Here's how the part is built. I have some questions about the finished solid (model axes, mm). Coordinates: 2 decimals unless noted, no trailing zeros. Loops run counter-clockwise (first coordinate to the right, second up) from the corner with the lowest first, then second, coordinate; pieces in that order, holes last. Notation, with made-up numbers: (58, 46) -> (111, 46) arc R28 cw to (111, 77) -> close; hole circle Ø10 at (-30, -6). An arc over 180 degrees is marked (long way). Answer as a JSON object with one key per item and string values. Group by question number.
Q1. I want a section at D-D on y = -15.5. Write out the boundary of the cut face in (x, z).
Q2. I want a section at B-B on x = 24.5. Write out the boundary of the cut face in (y, z).
Q3. I'm going to push flat-ended pins straight in: pin 1 (2 mm diameter, centred on y = -17.5, z = 25, fed in from +X); pin 2 (4 mm diameter, centred on x = 8.58, z = -35.9, fed in from +Y); pin 3 (1 mm diameter, centred on y = 17.5, z = 35, fed in from +X). Where does each tip first touch, or does it pass through?
Q4. I need wall thicknesses on line 1 (Y direction, x = 13.5, z = -23.5); line 2 (Z direction, x = 24.5, y = -21.95); line 3 (Z direction, x = 24, y = -23). Which ranges of each line are inside material? Lowest first, please.
Q5. I want a section at A-A on z = -25.9. Write out the boundary of the cut face in (x, y).
Q6. I want a section at C-C on z = 4.9. Write out the boundary of the cut face in (x, y).
```python
from build123d import *

# Parameters (mm, degrees)
SKETCH1_W                     = 120
SKETCH1_H                     = 50
BOSS_EXTRUDE1_DEPTH           = 34.5
SKETCH2_W                     = 71
SKETCH2_H                     = 5
CUT_EXTRUDE1_DEPTH            = 16
M4_CLEARANCE_HOLE1_D          = 4.5
M4_CLEARANCE_HOLE1_DEPTH      = 6
M4_CLEARANCE_HOLE2_AT_2_COUNT = 2
M4_CLEARANCE_HOLE2_AT_2_PITCH = 50.8
LPATTERN1_COUNT               = 4
LPATTERN1_PITCH               = 10
SKETCH9_W                     = 41
SKETCH9_H                     = 5
CUT_EXTRUDE2_DEPTH            = 16
CUT_EXTRUDE3_DEPTH            = 86.382960829
CHAMFER2_SIZE                 = 15
CHAMFER2_SIZE2                = 30
CHAMFER3_SIZE                 = 5


with BuildPart() as part:
    # Sketch1 → Boss-Extrude1 (new body)
    with BuildSketch(Plane(origin=(0, 0, 0), x_dir=(0, 0, -1), z_dir=(1, 0, 0))):
        Rectangle(SKETCH1_W, SKETCH1_H)
    extrude(amount=BOSS_EXTRUDE1_DEPTH)

    # Sketch2 → Cut-Extrude1 (cut)
    with BuildSketch(Plane(origin=(34.5, 0, 0), x_dir=(0, 0, -1), z_dir=(1, 0, 0))):
        with Locations((-19.5, -16.5)):
            Rectangle(SKETCH2_W, SKETCH2_H)
    extrude(amount=-CUT_EXTRUDE1_DEPTH, mode=Mode.SUBTRACT)

    # M4 Clearance Hole1
    with Locations(Plane(origin=(0, -25, 0), x_dir=(-1, 0, 0), z_dir=(0, -1, 0))):
        with Locations((-24.5, -50), (-24.5, 10)):
            Hole(M4_CLEARANCE_HOLE1_D / 2, depth=M4_CLEARANCE_HOLE1_DEPTH)

    # Sketch8 → M4 Clearance Hole2 (revolve, cut)
    with BuildSketch(Plane(origin=(8.58, 25, -15.9), x_dir=(0, 0, 1), z_dir=(1, 0, 0))):
        Polygon((0, 0), (0, 7.351936393), (2.25, 6), (2.25, 0), align=None)
    m4_clearance_hole2 = revolve(axis=Axis((8.58, 31.35, -15.9), (0, -1, 0)), mode=Mode.SUBTRACT)

    # M4 Clearance Hole2 at 2: M4 Clearance Hole2 ×2
    with Locations(*[(0, 0, i * M4_CLEARANCE_HOLE2_AT_2_PITCH) for i in range(1, M4_CLEARANCE_HOLE2_AT_2_COUNT)]):
        add(m4_clearance_hole2, mode=Mode.SUBTRACT)

    # LPattern1: M4 Clearance Hole2 ×4
    with Locations(*[(0, 0, -i * LPATTERN1_PITCH) for i in range(1, LPATTERN1_COUNT)]):
        add(m4_clearance_hole2, mode=Mode.SUBTRACT)

    # LPattern1 copy 1 sketch → LPattern1 copy 1 (revolve, cut)
    with BuildSketch(Plane(origin=(8.58, 25, 24.9), x_dir=(0, 0, 1), z_dir=(1, 0, 0))):
        Polygon((0, 0), (0, 7.351936393), (2.25, 6), (2.25, 0), align=None)
    revolve(axis=Axis((8.58, 31.35, 24.9), (0, -1, 0)), mode=Mode.SUBTRACT)

    # LPattern1 copy 2 sketch → LPattern1 copy 2 (revolve, cut)
    with BuildSketch(Plane(origin=(8.58, 25, 14.9), x_dir=(0, 0, 1), z_dir=(1, 0, 0))):
        Polygon((0, 0), (0, 7.351936393), (2.25, 6), (2.25, 0), align=None)
    revolve(axis=Axis((8.58, 31.35, 14.9), (0, -1, 0)), mode=Mode.SUBTRACT)

    # LPattern1 copy 3 sketch → LPattern1 copy 3 (revolve, cut)
    with BuildSketch(Plane(origin=(8.58, 25, 4.9), x_dir=(0, 0, 1), z_dir=(1, 0, 0))):
        Polygon((0, 0), (0, 7.351936393), (2.25, 6), (2.25, 0), align=None)
    revolve(axis=Axis((8.58, 31.35, 4.9), (0, -1, 0)), mode=Mode.SUBTRACT)

    # Sketch9 → Cut-Extrude2 (cut)
    with BuildSketch(Plane.ZY):
        with Locations((-30.9, 16.5)):
            Rectangle(SKETCH9_W, SKETCH9_H)
        with Locations((19.9, 16.5)):
            Rectangle(SKETCH9_W, SKETCH9_H)
    extrude(amount=-CUT_EXTRUDE2_DEPTH, mode=Mode.SUBTRACT)

    # Sketch10 → Cut-Extrude3 (cut, through all)
    with BuildSketch(Plane(origin=(0, 25, 0), x_dir=(1, 0, 0), z_dir=(0, 1, 0))):
        Polygon((34.5, 60), (15, 60), (34.5, 21), align=None)
    extrude(amount=-CUT_EXTRUDE3_DEPTH, mode=Mode.SUBTRACT)

    # Chamfer2
    chamfer2_edges = [part.edges().sort_by_distance(p)[0] for p in [
        (34.5, 25, 19.5),
    ]]
    chamfer2_side = [part.faces().sort_by_distance(p)[0] for p in [
        (16.428375325, 25, 5.112583766),
    ]]
    chamfer(chamfer2_edges, length=CHAMFER2_SIZE, length2=CHAMFER2_SIZE2, reference=chamfer2_side[0])

    # Chamfer3
    chamfer3_edges = [part.edges().sort_by_distance(p)[0] for p in [
        (7.5, 25, -60),
        (7.5, -25, -60),
        (9.75, 25, 60),
        (17.25, -25, 60),
    ]]
    chamfer(chamfer3_edges, length=CHAMFER3_SIZE)


solid = part.part
```
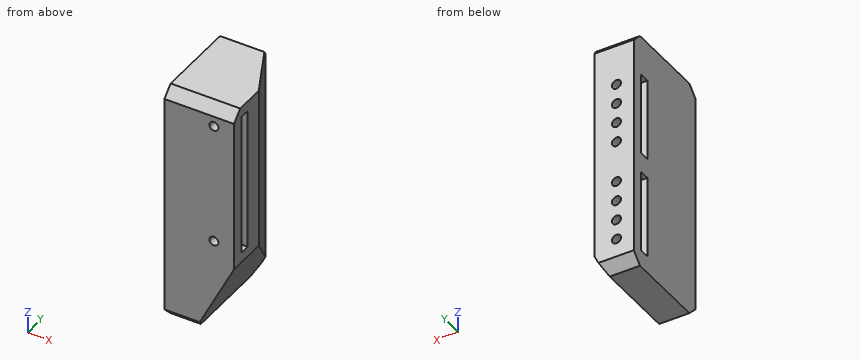
Result set:
{
 "1": {"outline": "(0, -60) -> (15, -60) -> (34.5, -21) -> (34.5, -16) -> (18.5, -16) -> (18.5, 55) -> (34.5, 55) -> (34.5, 60) -> (0, 60) -> close"},
 "2": {"outline": "(-25, -41) -> (15, -41) -> (15, 60) -> (-20, 60) -> (-25, 55) -> (-25, 52.25) -> (-19, 52.25) -> (-19, 55) -> (-14, 55) -> (-14, -16) -> (-19, -16) -> (-19, -12.25) -> (-25, -12.25) -> close; (-25, -7.75) -> (-19, -7.75) -> (-19, 47.75) -> (-25, 47.75) -> close"},
 "3": {"pin 1": "stops at x = 18.5", "pin 2": "stops at y = 14", "pin 3": "stops at x = 23.5"},
 "4": {"line 1": "y = -25 to 14, 19 to 25", "line 2": "z = -41 to -12.25, -7.75 to 47.75, 52.25 to 58.05", "line 3": "z = -42 to -12.19, -7.81 to 47.81, 52.19 to 57"},
 "5": {"outline": "(0, -25) -> (32.05, -25) -> (32.05, -0.1) -> (19.5, 25) -> (10.83, 25) -> (10.83, 19) -> (16, 19) -> (16, 14) -> (0, 14) -> close; (0, 19) -> (6.33, 19) -> (6.33, 25) -> (0, 25) -> close"},
 "6": {"outline": "(0, -25) -> (34.5, -25) -> (34.5, -19) -> (18.5, -19) -> (18.5, -14) -> (34.5, -14) -> (34.5, -5) -> (19.5, 25) -> (10.83, 25) -> (10.83, 19) -> (16, 19) -> (16, 14) -> (0, 14) -> close; (0, 19) -> (6.33, 19) -> (6.33, 25) -> (0, 25) -> close"}
}
